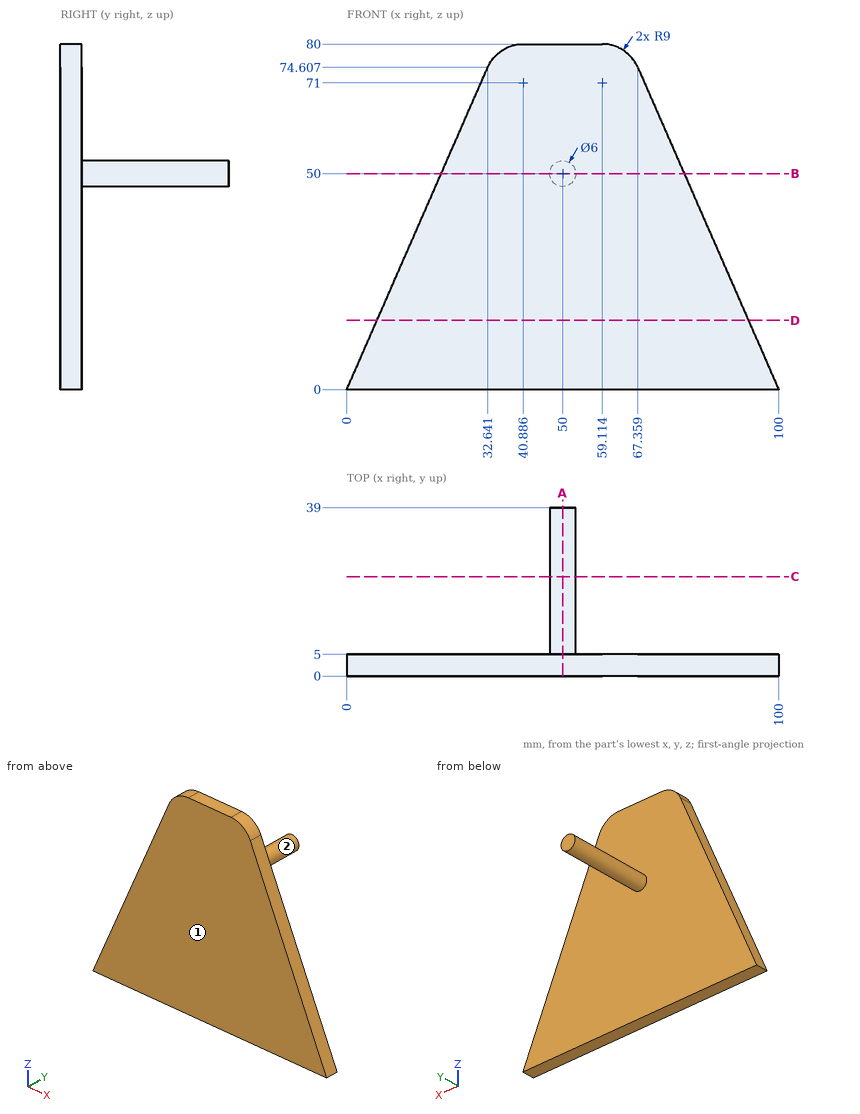
Geometry check sheet. Reference: drawing and pictorial views, mm from the part's lowest x, y, z. A direction names the side the tool comes from. Coordinates: 2 decimals unless noted, no trailing zeros. Write each loop counter-clockwise with the first axis right and the second up, starting at its lowest first coordinate (ties: lowest second). Pieces come first, ordered by that corner, then holes. Notation, with made-up numbers: (-17, 86) - (9, 86) arc R7 cw to (9, 94) - close; hole circle Ø9 at (2.25, 25.5). An arc over 180 degrees is marked (long way). One line per question, with ' | ' between items. Start each with the question number.
1. Section check B-B (z = 50). Enter the section's corners in (x, y) (1 decimal).
2. Material ranges on line 1 along Y through (x, z) = (25.5, 41); line 2 along Z through (x, y) = (76, 3.5) (1 decimal); line 3 along X through (y, z) = (3, 52), recorded low to high.
3. Access from +Z, -Z, +X, -X, +Y, -Y to the whole of each face (thin tool, end or side, straight path). Record for the marked faces 1 and 2.
4. Section check C-C (y = 23). Enter the section's corners in (x, z), plus the area to 3 significant figures.
5. Section check A-A (x = 50). Enter the section's corners in (y, z), plus the area to 3 significant figures.
6. Section check D-D (z = 16). Enter the section's corners in (x, y), plus the area to 3 significant figures.
Computed values:
1) outline: (21.9, 0) - (78.1, 0) - (78.1, 5) - (53, 5) - (53, 39) - (47, 39) - (47, 5) - (21.9, 5) - close
2) line 1: 0 to 5 | line 2: 0 to 54.9 | line 3: 22.75 to 77.25
3) face 1: +Z, -Z, +X, -X, -Y | face 2: +Y
4) outline: circle Ø6 at (50, 50) | area: 28.3 mm²
5) outline: (0, 0) - (5, 0) - (5, 47) - (39, 47) - (39, 53) - (5, 53) - (5, 80) - (0, 80) - close | area: 604 mm²
6) outline: (7, 0) - (93, 0) - (93, 5) - (7, 5) - close | area: 430 mm²
